```python
from build123d import *

# Parameters (mm, degrees)
SKETCH2_R               = 3.4925
BOSS_EXTRUDE1_DEPTH     = 101.6
FILLET1_R               = 2.54
SKETCH12_R              = 7.77875
CUT_EXTRUDE2_DEPTH      = 22.706691527
CUT_EXTRUDE2_DEPTH_BACK = 58.627716011
SKETCH13_R              = 7.77875
CUT_EXTRUDE3_DEPTH      = 22.706691527
CUT_EXTRUDE3_DEPTH_BACK = 58.627716011
SKETCH14_R              = 10.795
SKETCH14_R_2            = 7.77875
BOSS_EXTRUDE2_DEPTH     = 76.2
SKETCH14_2_R            = 7.77875
CUT_EXTRUDE4_DEPTH      = 102.6
BOSS_EXTRUDE3_DEPTH     = 25.4


with BuildPart() as part:
    # Sketch2 → Boss-Extrude1 (new body)
    with BuildSketch(Plane(origin=(0, 0, 0), x_dir=(1, 0, 0), z_dir=(0, 1, 0))):
        Polygon((19.05, -6.35), (31.75, -6.35), (31.75, 6.35), (19.05, 6.35), (0, 25.4), (-19.05, 6.35), (-31.75, 6.35), (-31.75, -6.35), (-19.05, -6.35), (0, -25.4), align=None)
        Polygon((-19.05, 2.757897552), (0, 21.807897552), (19.05, 2.757897552), (19.05, -2.757897552), (0, -21.807897552), (-19.05, -2.757897552), align=None, mode=Mode.SUBTRACT)
        with Locations((25.4, 0)):
            Circle(SKETCH2_R, mode=Mode.SUBTRACT)
        with Locations((-25.4, 0)):
            Circle(SKETCH2_R, mode=Mode.SUBTRACT)
    extrude(amount=BOSS_EXTRUDE1_DEPTH)

    # Fillet1
    fillet1_edges = [part.edges().sort_by_distance(p)[0] for p in [
        (0, 50.8, 25.4),
        (-19.05, 50.8, 6.35),
        (-31.75, 50.8, 6.35),
        (-31.75, 50.8, -6.35),
        (-19.05, 50.8, -6.35),
        (0, 50.8, -25.4),
        (19.05, 50.8, -6.35),
        (31.75, 50.8, -6.35),
        (31.75, 50.8, 6.35),
        (19.05, 50.8, 6.35),
    ]]
    fillet(fillet1_edges, radius=FILLET1_R)

    # Sketch12 → Cut-Extrude2 (cut, two sides)
    with BuildSketch(Plane(origin=(-12.7, 0, -12.7), x_dir=(-0.707106781, 0, 0.707106781), z_dir=(-0.707106781, 0, -0.707106781))) as cut_extrude2_sk:
        with Locations((0, 76.2)):
            Circle(SKETCH12_R)
    extrude(amount=CUT_EXTRUDE2_DEPTH, mode=Mode.SUBTRACT)
    extrude(cut_extrude2_sk.sketch, amount=-CUT_EXTRUDE2_DEPTH_BACK, mode=Mode.SUBTRACT)

    # Sketch13 → Cut-Extrude3 (cut, two sides)
    with BuildSketch(Plane(origin=(12.7, 0, -12.7), x_dir=(-0.707106781, 0, -0.707106781), z_dir=(0.707106781, 0, -0.707106781))) as cut_extrude3_sk:
        with Locations((0, 50.8)):
            Circle(SKETCH13_R)
    extrude(amount=CUT_EXTRUDE3_DEPTH, mode=Mode.SUBTRACT)
    extrude(cut_extrude3_sk.sketch, amount=-CUT_EXTRUDE3_DEPTH_BACK, mode=Mode.SUBTRACT)

    # Sketch14 → Boss-Extrude2 (add)
    with BuildSketch(Plane.XZ):
        with Locations((0, 28.157897552)):
            Circle(SKETCH14_R)
        with Locations((0, 28.157897552)):
            Circle(SKETCH14_R_2, mode=Mode.SUBTRACT)
    extrude(amount=-BOSS_EXTRUDE2_DEPTH)

    # Sketch14<2> → Cut-Extrude4 (cut, through all)
    with BuildSketch(Plane.XZ):
        with Locations((0, 28.157897552)):
            Circle(SKETCH14_2_R)
    extrude(amount=-CUT_EXTRUDE4_DEPTH, mode=Mode.SUBTRACT)

    # Sketch15 → Boss-Extrude3 (add)
    with BuildSketch(Plane(origin=(0, 76.2, 0), x_dir=(1, 0, 0), z_dir=(0, 1, 0))):
        with BuildLine():
            Line((1.316531006, -20.491366545), (3.766569527, -18.041328024))
            ThreePointArc((3.766569527, -18.041328024), (0, -17.362897552), (-3.766569527, -18.041328024))
            Line((-3.766569527, -18.041328024), (-1.316531006, -20.491366545))
            ThreePointArc((-1.316531006, -20.491366545), (0, -20.379147552), (1.316531006, -20.491366545))
        make_face()
    extrude(amount=BOSS_EXTRUDE3_DEPTH)


solid = part.part
```
Check sheet for the modelled part. Datum: model origin and axes. Units: mm. A direction names the side the tool comes from. Round coordinates to 2 decimals unless told otherwise and drop trailing zeros. Order: outer loops, then holes, each group sorted by start corner. A loop starts at its lowest first (then second) coordinate and runs counter-clockwise, first axis right, second up.
1) Mould release check, pull along Z, two halves, no side actions. Record for faces 1 (the flat face through (11.52, 50.09, 10.29)), 2 (the cylindrical face through (-30.986, 51.511, 5.626)), 3 (the flat face through (9, 0, 14)): +Z half, -Z half, draft (parallel to the pull), parting line (faces both ways), or undercut.
2) Go/stop test with flat-tipped pins: pin 1 Ø15.5 at (x, z) = (2.5, 31.5) entering from +Y; pin 2 Ø2 at (y, z) = (12.5, 5) entering from -X; pin 3 Ø6 at (x, y) = (-14, 30.5) entering from +Z. Record where each tip stops, or that it passes through.
3) Section check B-B (x = 25.4). Record the boundary of the cut face in (y, z).
4) Section check A-A (z = 0). Record the boundary of the cut face in (x, y).
5) Tool access check on faces 4 (the flat face through (-25, 50, -6.35)), 5 (the flat face through (-19.05, 50, 0)), 6 (the flat face through (-25, 50, 6.35)). Record the directions out of +Z, -Z, +X, -X, +Y, -Y that give a thin tool (end or side, any length) a straight path to the whole face; none if there is none.
6) Scan lines: line 1 (Z direction, x = 0, y = 50); line 2 (X direction, y = 63, z = 0); line 3 (Z direction, x = -25.4, y = 59). Record each from-to range of solid material in increasing order.
7) Section check C-C (y = 9.5). Give the number of separate pieces and of enclosed holes in the cut face, and give its area (3 significant figures).
8) Section check D-D (z = 28). Record the boundary of the cut face in (x, y), and give its area (3 significant figures).
Result:
1. face 1: undercut
1. face 2: +Z half
1. face 3: draft
2. pin 1: stops at y = 76.2
2. pin 2: stops at x = -31.74
2. pin 3: stops at z = 14.4
3. outline: (0, -6.35) - (101.6, -6.35) - (101.6, -3.49) - (0, -3.49) - close; (0, 3.49) - (101.6, 3.49) - (101.6, 6.35) - (0, 6.35) - close
4. outline: (-31.75, 0) - (-28.89, 0) - (-28.89, 101.6) - (-31.75, 101.6) - close; (-21.91, 0) - (-19.05, 0) - (-19.05, 101.6) - (-21.91, 101.6) - close; (19.05, 0) - (21.91, 0) - (21.91, 101.6) - (19.05, 101.6) - close; (28.89, 0) - (31.75, 0) - (31.75, 101.6) - (28.89, 101.6) - close
5. face 4: -Z, -X, +Y, -Y
5. face 5: +Y, -Y
5. face 6: +Z, -X, +Y, -Y
6. line 1: z = -24.35 to -21.81, 17.36 to 20.38, 35.94 to 38.95
6. line 2: x = -31.75 to -28.89, -21.91 to -19.05, 19.05 to 21.91, 28.89 to 31.75
6. line 3: z = -6.35 to -3.49, 3.49 to 6.35
7. separate pieces: 1
7. enclosed holes: 4
7. area: 653 mm2
8. outline: (-10.79, 0) - (-7.78, 0) - (-7.78, 76.2) - (-10.79, 76.2) - close; (7.78, 0) - (10.79, 0) - (10.79, 76.2) - (7.78, 76.2) - close
8. area: 460 mm2
